Could you check a few things on this model? Use its own coordinates, in mm. A direction names the side the tool comes from. Give positions to 0.01 mm unless a question says otherwise; leave off trailing zeros. Loops run counter-clockwise (first coordinate to the right, second up) from the corner with the lowest first, then second, coordinate; pieces in that order, holes last. Notation, with made-up numbers: M -39.75,-7.5 L 18.25,-7.5 A6 ccw 18.25,1.5 Z; hole C 66.5,0.5 d11. An arc over 180 degrees is marked long. Use a Markdown table: item, result. Add a question column.
1) Will these pins go through, and if not, where does the flat tip stop? pin 1 Ø0.7 at (x, z) = (-63.5, 1.5) entering from +Y; pin 2 Ø1.4 at (x, z) = (-26, 1) entering from -Y; pin 3 Ø0.6 at (x, z) = (-14, 0.5) entering from +Y.
2) We'd pull the mould along Y, two halves only. Please class faces 6 (the flat face through (-32, 0, 0.5)), 7 (the flat face through (-37, 10, 1)), 8 (the flat face through (-14, 4, 0)): +Y half, -Y half, draft (parallel to the pull), parting line (faces both ways), or undercut.
3) Suppose I cut it at B-B on x = -11.5. List the corners of the cut face in (y, z) for me, and give its area (3 significant figures).
4) Which directions (+Z, -Z, +X, -X, +Y, -Y) give clear straight access to the entire face, cutting with the end or side of a thin tool? Please do faces 1 (the flat face through (-63, -0.5, 2)), 2 (the flat face through (-25.5, 7, 1.3)), 3 (the flat face through (20, 0, 1)), 4 (the flat face through (0, -9, 1)), 5 (the flat face through (-65.2, -2, 1)).
5) Suppose I cut it at A-A on y = 9. List the corners of the cut face in (x, z) for me, and give its area (3 significant figures).
6) If I drill on line 1 along Y through (x, z) = (-61, 0.85); line 2 along Y through (x, z) = (-41, 0.15); line 3 along X through (y, z) = (-9.5, 0.55), over which ranges is the centre line in solid material (lowest first)? Write a range as [from, to].
7) Suppose I cut it at D-D on y = -7.5. List the corners of the cut face in (x, z) for me.
8) Suppose I cut it at C-C on z = 2.25. List the corners of the cut face in (x, y) for me.
```python
from build123d import *

# Parameters (mm, degrees)
BOSS_EXTRUDE1_DEPTH = 2.7
CUT_EXTRUDE1_START  = -2.7
SKETCH2_W           = 68.2
SKETCH2_H           = 1.4
CUT_EXTRUDE1_DEPTH  = 0.5


with BuildPart() as part:
    # Sketch1 → Boss-Extrude1 (new body)
    with BuildSketch(Plane.XY):
        Polygon((20, 15), (0, 15), (0, 8), (-15.5, 8), (-19.5, 6), (-23.5, 6), (-27.5, 8), (-31.5, 8), (-35.5, 10), (-39.5, 10), (-43.5, 8), (-47.5, 8), (-60.25, -0.5), (-65.2, -0.5), (-65.2, -4), (0, -4), (0, -15), (20, -15), align=None)
    extrude(amount=BOSS_EXTRUDE1_DEPTH)

    # Sketch2 → Cut-Extrude1 (cut)
    with BuildSketch(Plane.XY.offset(2.7).offset(CUT_EXTRUDE1_START)):
        with Locations((-31.1, -0.5)):
            Rectangle(SKETCH2_W, SKETCH2_H)
    extrude(amount=CUT_EXTRUDE1_DEPTH, mode=Mode.SUBTRACT)


solid = part.part
```
Answer block:
| question | item | result |
|---|---|---|
| 1 | pin 1 | stops at y = -0.5 |
| 1 | pin 2 | stops at y = -4 |
| 1 | pin 3 | stops at y = 8 |
| 2 | face 6 | undercut |
| 2 | face 7 | +Y half |
| 2 | face 8 | draft |
| 3 | outline | M -4,0 L -1.2,0 L -1.2,0.5 L 0.2,0.5 L 0.2,0 L 8,0 L 8,2.7 L -4,2.7 Z |
| 3 | area | 31.7 mm^2 |
| 4 | face 1 | +Z, -Z, -X, +Y |
| 4 | face 2 | +Z, -Z, +Y |
| 4 | face 3 | +Z, -Z, +X, +Y, -Y |
| 4 | face 4 | +Z, -Z, -X, -Y |
| 4 | face 5 | +Z, -Z, -X, +Y, -Y |
| 5 | outline | M -41.5,0 L -33.5,0 L -33.5,2.7 L -41.5,2.7 Z; M 0,0 L 20,0 L 20,2.7 L 0,2.7 Z |
| 5 | area | 75.6 mm^2 |
| 6 | line 1 | y = [-4, -0.5] |
| 6 | line 2 | y = [-4, -1.2], [0.2, 9.25] |
| 6 | line 3 | x = [0, 20] |
| 7 | outline | M 0,0 L 20,0 L 20,2.7 L 0,2.7 Z |
| 8 | outline | M -65.2,-4 L 0,-4 L 0,-15 L 20,-15 L 20,15 L 0,15 L 0,8 L -15.5,8 L -19.5,6 L -23.5,6 L -27.5,8 L -31.5,8 L -35.5,10 L -39.5,10 L -43.5,8 L -47.5,8 L -60.25,-0.5 L -65.2,-0.5 Z |
